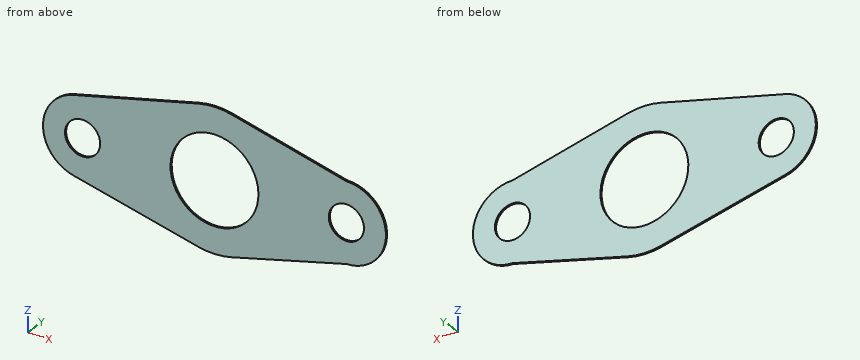
```python
from build123d import *

# Parameters (mm, degrees)
SKETCH1_R           = 22.5
SKETCH1_R_2         = 10
SKETCH1_R_3         = 40
SKETCH1_R_4         = 25
BOSS_EXTRUDE1_DEPTH = 1


with BuildPart() as part:
    # Sketch1 → Boss-Extrude1 (new body)
    # profile 1 of 5: a face of its own
    with BuildSketch(Plane(origin=(0, 0, 0), x_dir=(1, 0, 0), z_dir=(0, 1, 0))):
        with Locations((-75, 0)):
            Circle(SKETCH1_R)
        with Locations(Location((-75, 0, 0), (0, 0, 270))):
            Circle(SKETCH1_R_2, mode=Mode.SUBTRACT)
    # profile 2 of 5: a face of its own
    with BuildSketch(Plane(origin=(0, 0, 0), x_dir=(1, 0, 0), z_dir=(0, 1, 0))):
        with BuildLine():
            ThreePointArc((-52.5, 0), (-61.069368284, -17.668828484), (-80.25, -21.878928219))
            Line((-80.25, -21.878928219), (-9.333333333, -38.895872389))
            ThreePointArc((-9.333333333, -38.895872389), (-40, 0), (-9.333333333, 38.895872389))
            Line((-9.333333333, 38.895872389), (-80.25, 21.878928219))
            ThreePointArc((-80.25, 21.878928219), (-61.069368284, 17.668828484), (-52.5, 0))
        make_face()
    # profile 3 of 5: a face of its own
    with BuildSketch(Plane(origin=(0, 0, 0), x_dir=(1, 0, 0), z_dir=(0, 1, 0))):
        Circle(SKETCH1_R_3)
        with Locations(Location((0, 0, 0), (0, 0, 270))):
            Circle(SKETCH1_R_4, mode=Mode.SUBTRACT)
    # profile 4 of 5: a face of its own
    with BuildSketch(Plane(origin=(0, 0, 0), x_dir=(1, 0, 0), z_dir=(0, 1, 0))):
        with BuildLine():
            ThreePointArc((40, 0), (31.524856574, -24.620792392), (9.6908291, -38.808347444))
            Line((9.6908291, -38.808347444), (75, -22.5))
            ThreePointArc((75, -22.5), (52.5, 0), (75, 22.5))
            Line((75, 22.5), (9.6908291, 38.808347444))
            ThreePointArc((9.6908291, 38.808347444), (31.524856574, 24.620792392), (40, 0))
        make_face()
    # profile 5 of 5: a face of its own
    with BuildSketch(Plane(origin=(0, 0, 0), x_dir=(1, 0, 0), z_dir=(0, 1, 0))):
        with Locations((75, 0)):
            Circle(SKETCH1_R)
        with Locations(Location((75, 0, 0), (0, 0, 270))):
            Circle(SKETCH1_R_2, mode=Mode.SUBTRACT)
    extrude(amount=BOSS_EXTRUDE1_DEPTH)


solid = part.part
```
CAD build for the part. Positions are in the model's coordinates, mm. Round coordinates to 2 decimals unless told otherwise and drop trailing zeros. Loops run counter-clockwise (first coordinate to the right, second up) from the corner with the lowest first, then second, coordinate; pieces in that order, holes last. Notation, with made-up numbers: M -4,-18 L 2,-18 A32 ccw 2,15 Z; hole C -23.5,27.5 d3. An arc over 180 degrees is marked long. Use a Markdown table: item, result. Add a question column.
(1) Cut at C-C (x = 0). Give the cut face in (y, z), and give its area (3 significant figures).
(2) Flat gauge pin, fed straight in: pin 1 (18 mm diameter, centred on x = -75, z = 0, fed in from +Y). Where does the tip first touch, or does it go through?
(3) Cut at A-A (z = 0). Give the cut face in (x, y).
(4) Cut at B-B (y = 0.8). Give the cut face in (x, z).
(5) Cut at D-D (z = -16.5). Give the cut face in (x, y), and give its area (3 significant figures).
(6) Drill centre lines: line 1 (X direction, y = 0.6, z = 3.5); line 2 (X direction, y = 0.2, z = 6); line 3 (X direction, y = 0.9, z = 11). Where is each one in solid material? Low to high.
Geometry says:
| question | item | result |
|---|---|---|
| 1 | outline | M 0,-40 L 1,-40 L 1,-25 L 0,-25 Z; M 0,25 L 1,25 L 1,40 L 0,40 Z |
| 1 | area | 30.0 mm² |
| 2 | pin 1 | passes through |
| 3 | outline | M -97.5,0 L -85,0 L -85,1 L -97.5,1 Z; M -65,0 L -25,0 L -25,1 L -65,1 Z; M 25,0 L 65,0 L 65,1 L 25,1 Z; M 85,0 L 97.5,0 L 97.5,1 L 85,1 Z |
| 4 | outline | M -80.25,-21.88 L -9.33,-38.9 A40 ccw 9.69,-38.81 L 75,-22.5 A22.5 ccw 75,22.5 L 9.69,38.81 A40 ccw -9.33,38.9 L -80.25,21.88 A22.5 ccw Z; hole C -75,0 d20; hole C 0,0 d50; hole C 75,0 d20 |
| 5 | outline | M -90.3,0 L -18.78,0 L -18.78,1 L -90.3,1 Z; M 18.78,0 L 90.3,0 L 90.3,1 L 18.78,1 Z |
| 5 | area | 143 mm² |
| 6 | line 1 | x = -97.23 to -84.37, -65.63 to -24.75, 24.75 to 65.63, 84.37 to 97.23 |
| 6 | line 2 | x = -96.69 to -83, -67 to -24.27, 24.27 to 67, 83 to 96.69 |
| 6 | line 3 | x = -94.63 to -22.45, 22.45 to 94.63 |
